The drawing under review shows one solid part. Ordinate dimensions are in mm from its lowest x, y, z. Coordinates: 2 decimals unless noted, no trailing zeros. Write each loop counter-clockwise with the first axis right and the second up, starting at its lowest first coordinate (ties: lowest second). Pieces come first, ordered by that corner, then holes.
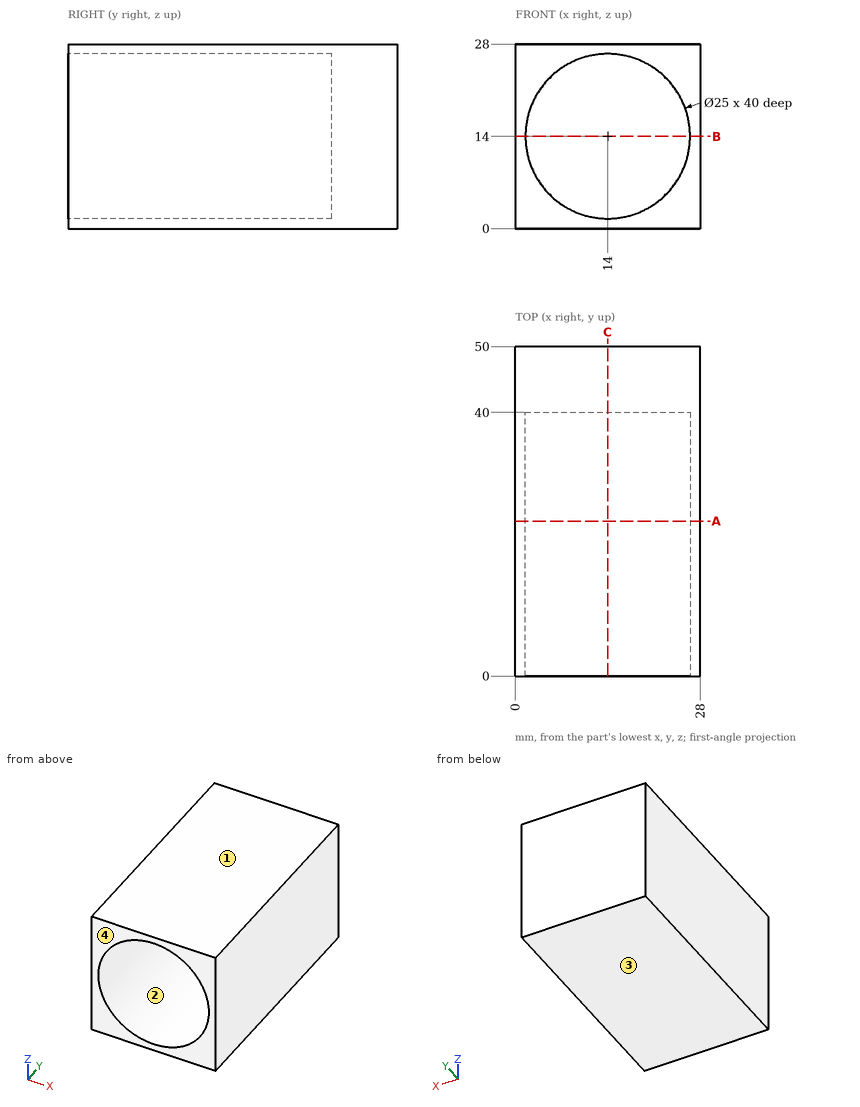
Q1. For probe 1 along X at (y, z) = (22, 14); probe 2 along Y at (x, z) = (21.5, 20.75), list the stretches that pass through material, from the lowest coordinate up.
Ans:
probe 1: x = 0 to 1.5, 26.5 to 28
probe 2: y = 40 to 50
Q2. Add section A-A (y = 23.5). State the section outline as (x, z) points, then the cut area to 3 significant figures.
Ans:
outline: (0, 0) - (28, 0) - (28, 28) - (0, 28) - close; hole circle Ø25 at (14, 14)
area: 293 mm2
Q3. Add section C-C (x = 14). State the section outline as (y, z) points.
Ans:
outline: (0, 0) - (50, 0) - (50, 28) - (0, 28) - (0, 26.5) - (40, 26.5) - (40, 1.5) - (0, 1.5) - close
Q4. Draft analysis for pull direction Z (two halves, no side actions). For the marked faces 1, 2, 3 and 4, state which applies: +Z half, -Z half, draft (parallel to the pull), parting line (faces both ways), or undercut.
Ans:
face 1: +Z half
face 2: undercut
face 3: -Z half
face 4: draft
Q5. Clearance check with flat-ended pins moving along their axes: pin 1 Ø2 at (y, z) = (37.5, 8) entering from -X; pin 2 Ø7.5 at (x, z) = (8, 9) entering from -Y. State where each tip first meets the part, or that it passes through.
Ans:
pin 1: stops at x = 0
pin 2: stops at y = 40
Q6. Add section B-B (z = 14). State the section outline as (x, y) points.
Ans:
outline: (0, 0) - (1.5, 0) - (1.5, 40) - (26.5, 40) - (26.5, 0) - (28, 0) - (28, 50) - (0, 50) - close
